from build123d import *

# Parameters (mm, degrees)
SKETCH1_W           = 88.9
SKETCH1_H           = 31.75
BOSS_EXTRUDE1_DEPTH = 3.175
CUT_EXTRUDE1_REACH  = 49.625
SKETCH2_R           = 1.63195
SKETCH2_R_2         = 6.35


with BuildPart() as part:
    # Sketch1 → Boss-Extrude1 (new, symmetric)
    with BuildSketch(Plane(origin=(0, 0, 0), x_dir=(0, 0, -1), z_dir=(1, 0, 0))):
        Rectangle(SKETCH1_W, SKETCH1_H)
    extrude(amount=BOSS_EXTRUDE1_DEPTH, both=True)

    # Sketch2 → Cut-Extrude1 (cut, up to next)
    with BuildSketch(Plane(origin=(3.175, 0, 0), x_dir=(0, 0, -1), z_dir=(1, 0, 0)), mode=Mode.PRIVATE) as cut_extrude1_sk1:
        with Locations((-23.114, 8.255)):
            Circle(SKETCH2_R)
    cut_extrude1_tool1 = extrude(cut_extrude1_sk1.sketch, amount=-CUT_EXTRUDE1_REACH, mode=Mode.PRIVATE) & part.part
    # Sketch2 → Cut-Extrude1 (cut, up to next)
    with BuildSketch(Plane(origin=(3.175, 0, 0), x_dir=(0, 0, -1), z_dir=(1, 0, 0)), mode=Mode.PRIVATE) as cut_extrude1_sk2:
        with Locations((-23.114, -12.7)):
            Circle(SKETCH2_R)
    cut_extrude1_tool2 = extrude(cut_extrude1_sk2.sketch, amount=-CUT_EXTRUDE1_REACH, mode=Mode.PRIVATE) & part.part
    # Sketch2 → Cut-Extrude1 (cut, up to next)
    with BuildSketch(Plane(origin=(3.175, 0, 0), x_dir=(0, 0, -1), z_dir=(1, 0, 0)), mode=Mode.PRIVATE) as cut_extrude1_sk3:
        with Locations((33.655, -12.7)):
            Circle(SKETCH2_R)
    cut_extrude1_tool3 = extrude(cut_extrude1_sk3.sketch, amount=-CUT_EXTRUDE1_REACH, mode=Mode.PRIVATE) & part.part
    # Sketch2 → Cut-Extrude1 (cut, up to next)
    with BuildSketch(Plane(origin=(3.175, 0, 0), x_dir=(0, 0, -1), z_dir=(1, 0, 0)), mode=Mode.PRIVATE) as cut_extrude1_sk4:
        with Locations((33.655, 8.255)):
            Circle(SKETCH2_R)
    cut_extrude1_tool4 = extrude(cut_extrude1_sk4.sketch, amount=-CUT_EXTRUDE1_REACH, mode=Mode.PRIVATE) & part.part
    # Sketch2 → Cut-Extrude1 (cut, up to next)
    with BuildSketch(Plane(origin=(3.175, 0, 0), x_dir=(0, 0, -1), z_dir=(1, 0, 0)), mode=Mode.PRIVATE) as cut_extrude1_sk5:
        with Locations((-10.414, -2.2225)):
            Circle(SKETCH2_R_2)
    cut_extrude1_tool5 = extrude(cut_extrude1_sk5.sketch, amount=-CUT_EXTRUDE1_REACH, mode=Mode.PRIVATE) & part.part
    add(cut_extrude1_tool1.solids().sort_by_distance((3.175, 8.255, 23.114))[0], mode=Mode.SUBTRACT)
    add(cut_extrude1_tool2.solids().sort_by_distance((3.175, -12.7, 23.114))[0], mode=Mode.SUBTRACT)
    add(cut_extrude1_tool3.solids().sort_by_distance((3.175, -12.7, -33.655))[0], mode=Mode.SUBTRACT)
    add(cut_extrude1_tool4.solids().sort_by_distance((3.175, 8.255, -33.655))[0], mode=Mode.SUBTRACT)
    add(cut_extrude1_tool5.solids().sort_by_distance((3.175, -2.2225, 10.414))[0], mode=Mode.SUBTRACT)


solid = part.part
Work out the finished part from the listing and answer in its coordinate system (mm). Coordinates: 2 decimals unless noted, no trailing zeros. Order: outer loops, then holes, each group sorted by start corner. A loop starts at its lowest first (then second) coordinate and runs counter-clockwise, first axis right, second up. Notation, with made-up numbers: (9.25, 51.25) - (31.25, 51.25) arc R30 cw to (31.25, 80.25) - close; hole circle Ø5 at (71, 29). An arc over 180 degrees is marked (long way). Put each result on its own line as item: value. Start each with the question number.
1) For a pull along Z with two mould halves and no side action, classify faces 1 (the flat face through (3.175, 0, 1)), 2 (the cylindrical face through (0.044, 6.807, 22.361)), 3 (the flat face through (0, 0, -44.45)) as released by +Z, released by -Z, zero draft, split by the parting line, or undercut.
2) Find section C-C (x = -1.25). State how many separate pieces and enclosed holes the cut face has, plus the area to 3 significant figures.
3) Find the intervals of material crossed by line 1 (Z direction, x = -1.5, y = -12.5); line 2 (Y direction, x = 1.5, z = -33) (3 decimals); line 3 (Y direction, x = -2, z = 7) (3 decimals), in increasing order. Write a range as from..to.
4) Find section A-A (y = -12.7). Give the vertices of the cut face in (x, z) (3 decimals).
5) Find section B-B (z = 6). Give the vertices of the cut face in (x, y) (3 decimals).
Results list:
1. face 1: zero draft
1. face 2: undercut
1. face 3: released by -Z
2. separate pieces: 1
2. enclosed holes: 5
2. area: 2,660 mm^2
3. line 1: z = -44.45..-35.27, -32.04..21.49, 24.73..44.45
3. line 2: y = -15.875..-14.195, -11.205..6.76, 9.75..15.875
3. line 3: y = -15.875..-7.577, 3.132..15.875
4. outline: (-3.175, -44.45) - (3.175, -44.45) - (3.175, -35.287) - (-3.175, -35.287) - close; (-3.175, -32.023) - (3.175, -32.023) - (3.175, 21.482) - (-3.175, 21.482) - close; (-3.175, 24.746) - (3.175, 24.746) - (3.175, 44.45) - (-3.175, 44.45) - close
5. outline: (-3.175, -15.875) - (3.175, -15.875) - (3.175, -6.787) - (-3.175, -6.787) - close; (-3.175, 2.342) - (3.175, 2.342) - (3.175, 15.875) - (-3.175, 15.875) - close
